```python
from build123d import *

# Parameters (mm, degrees)
SKETCH1_R           = 50
BOSS_EXTRUDE1_DEPTH = 10
SKETCH2_R           = 20
CUT_EXTRUDE1_DEPTH  = 74.484692283
CUT_EXTRUDE2_DEPTH  = 10
CUT_EXTRUDE3_DEPTH  = 10
CIRPATTERN1_COUNT   = 6
CIRPATTERN2_COUNT   = 6


with BuildPart() as part:
    # Sketch1 → Boss-Extrude1 (new, symmetric)
    with BuildSketch(Plane(origin=(0, 0, 0), x_dir=(1, 0, 0), z_dir=(0, 1, 0))):
        with Locations(Location((0, 0, 0), (0, 0, 270))):
            Circle(SKETCH1_R)
    extrude(amount=BOSS_EXTRUDE1_DEPTH, both=True)

    # Sketch2 → Cut-Extrude1 (cut, through all)
    with BuildSketch(Plane(origin=(0, 10, 0), x_dir=(1, 0, 0), z_dir=(0, 1, 0))):
        with Locations(Location((0, 0, 0), (0, 0, 270))):
            Circle(SKETCH2_R)
    extrude(amount=-CUT_EXTRUDE1_DEPTH, mode=Mode.SUBTRACT)

    # Sketch3 → Cut-Extrude2 (cut)
    with BuildSketch(Plane(origin=(0, 10, 0), x_dir=(1, 0, 0), z_dir=(0, 1, 0))):
        with BuildLine():
            Line((-7.5, 49.434299833), (-7.5, 18.540496218))
            ThreePointArc((-7.5, 18.540496218), (0, 20), (7.5, 18.540496218))
            Line((7.5, 18.540496218), (7.5, 49.434299833))
            ThreePointArc((7.5, 49.434299833), (0, 50), (-7.5, 49.434299833))
        make_face()
        with BuildLine():
            Line((39.061359474, 31.212340445), (12.306540723, 15.765438637))
            ThreePointArc((12.306540723, 15.765438637), (17.320508076, 10), (19.806540723, 2.77505758))
            Line((19.806540723, 2.77505758), (46.561359474, 18.221959388))
            ThreePointArc((46.561359474, 18.221959388), (43.301270189, 25), (39.061359474, 31.212340445))
        make_face()
        with BuildLine():
            Line((46.561359474, -18.221959388), (19.806540723, -2.77505758))
            ThreePointArc((19.806540723, -2.77505758), (17.320508076, -10), (12.306540723, -15.765438637))
            Line((12.306540723, -15.765438637), (39.061359474, -31.212340445))
            ThreePointArc((39.061359474, -31.212340445), (43.301270189, -25), (46.561359474, -18.221959388))
        make_face()
        with BuildLine():
            Line((7.5, -49.434299833), (7.5, -18.540496218))
            ThreePointArc((7.5, -18.540496218), (0, -20), (-7.5, -18.540496218))
            Line((-7.5, -18.540496218), (-7.5, -49.434299833))
            ThreePointArc((-7.5, -49.434299833), (0, -50), (7.5, -49.434299833))
        make_face()
        with BuildLine():
            Line((-39.061359474, -31.212340445), (-12.306540723, -15.765438637))
            ThreePointArc((-12.306540723, -15.765438637), (-17.320508076, -10), (-19.806540723, -2.77505758))
            Line((-19.806540723, -2.77505758), (-46.561359474, -18.221959388))
            ThreePointArc((-46.561359474, -18.221959388), (-43.301270189, -25), (-39.061359474, -31.212340445))
        make_face()
        with BuildLine():
            Line((-46.561359474, 18.221959388), (-19.806540723, 2.77505758))
            ThreePointArc((-19.806540723, 2.77505758), (-17.320508076, 10), (-12.306540723, 15.765438637))
            Line((-12.306540723, 15.765438637), (-39.061359474, 31.212340445))
            ThreePointArc((-39.061359474, 31.212340445), (-43.301270189, 25), (-46.561359474, 18.221959388))
        make_face()
    extrude(amount=-CUT_EXTRUDE2_DEPTH, mode=Mode.SUBTRACT)

    # Sketch4 → Cut-Extrude3 (cut)
    with BuildSketch(Plane(origin=(0, 10, 0), x_dir=(1, 0, 0), z_dir=(0, 1, 0))):
        with BuildLine():
            ThreePointArc((11, 48.774993593), (17.480362162, 30.322218565), (36.696416757, 33.961345633))
            ThreePointArc((36.696416757, 33.961345633), (24.971945946, 43.317455092), (11, 48.774993593))
        make_face()
    cut_extrude3 = extrude(amount=-CUT_EXTRUDE3_DEPTH, mode=Mode.SUBTRACT)

    # Sketch6 → Tap Drill for M10x1.0 Tap1 (revolve, cut)
    with BuildSketch(Plane(origin=(30, 10, 0), x_dir=(0, 0, 1), z_dir=(1, 0, 0))):
        Polygon((0, 0), (0, 72.703872786), (4.5, 70), (4.5, 0.025), (4.525, 0), align=None)
    tap_drill_for_m10x1_0_tap1 = revolve(axis=Axis((30, 16.35, 0), (0, -1, 0)), mode=Mode.SUBTRACT)

    # CirPattern1: Tap Drill for M10x1.0 Tap1 ×6 about axis
    cirpattern1_axis = Axis((0, 0, 0), (0, 1, 0))
    for i in range(1, CIRPATTERN1_COUNT):
        add(tap_drill_for_m10x1_0_tap1.rotate(cirpattern1_axis, i * 360 / CIRPATTERN1_COUNT), mode=Mode.SUBTRACT)

    # CirPattern2: Cut-Extrude3 ×6 about axis
    cirpattern2_axis = Axis((0, 0, 0), (0, 1, 0))
    for i in range(1, CIRPATTERN2_COUNT):
        add(cut_extrude3.rotate(cirpattern2_axis, i * 360 / CIRPATTERN2_COUNT), mode=Mode.SUBTRACT)


solid = part.part
```
Could you check a few things on this model? Use its own coordinates, in mm. A direction names the side the tool comes from. Coordinates: 2 decimals unless noted, no trailing zeros. Write each loop counter-clockwise with the first axis right and the second up, starting at its lowest first coordinate (ties: lowest second). Pieces come first, ordered by that corner, then holes. Notation, with made-up numbers: (50.25, 10) - (65.25, 10) arc R14 ccw to (65.25, 17) - close; hole circle Ø8 at (65.25, -2.5). An arc over 180 degrees is marked (long way). Use a Markdown table: item, result.
Q1. Thinking about a two-plate mould opening in X: for faces 4 (the cylindrical face through (-35, 5, 0)), 5 (the flat face through (23, 0, 37)), 6 (the cylindrical face through (17.779, 5.07, 30.153)), 7 (the flat face through (-20, 10, 29)), which applies, +X half, -X half, draft (parallel to the pull), parting line (faces both ways), or undercut?
Geometry check:
| item | result |
|---|---|
| face 4 | -X half |
| face 5 | undercut |
| face 6 | undercut |
| face 7 | draft |
Q2. Please list where these lines run through material, in increasing order: L1, parallel to X at y = -2.5, z = 0; L2, parallel to X at y = 8.25, z = -0.5; L3, parallel to Y at x = 2, z = 20.
Geometry check:
| item | result |
|---|---|
| L1 | x = -50 to -34.5, -25.5 to -20, 20 to 25.5, 34.5 to 50 |
| L2 | x = -35.01 to -34.47, -25.53 to -19.99, 19.99 to 25.53, 34.47 to 35.01 |
| L3 | y = -10 to 0 |
Q3. Imagine slicing it at B-B (z = -10). List the corners of the cut face in (x, y) for me, and give its area (3 significant figures).
Geometry check:
| item | result |
|---|---|
| outline | (-48.99, -10) - (-17.32, -10) - (-17.32, 0) - (-32.32, 0) - (-32.32, 10) - (-38.85, 10) - (-38.85, 0) - (-48.99, 0) - close; (17.32, -10) - (48.99, -10) - (48.99, 0) - (38.79, 0) - (38.79, 10) - (32.32, 10) - (32.32, 0) - (17.32, 0) - close |
| area | 763 mm2 |
Q4. Imagine slicing it at D-D (y = -3). List the corners of the cut face in (x, z) for me, and give its area (3 significant figures).
Geometry check:
| item | result |
|---|---|
| outline | circle Ø100 at (0, 0); hole circle Ø9 at (-30, 0); hole circle Ø40 at (0, 0); hole circle Ø9 at (-15, -25.98); hole circle Ø9 at (-15, 25.98); hole circle Ø9 at (15, -25.98); hole circle Ø9 at (15, 25.98); hole circle Ø9 at (30, 0) |
| area | 6,220 mm2 |
Q5. I'm going to push flat-ended pins straight in: pin 1 Ø2 at (x, z) = (-31.5, 4) entering from -Y; pin 2 Ø12 at (y, z) = (-3, -29) entering from -X; pin 3 Ø16.5 at (x, z) = (-18.5, 42) entering from +Y; pin 4 Ø5 at (y, z) = (3.5, -41) entering from -X. Where does each tip first touch, or does it pass through?
Geometry check:
| item | result |
|---|---|
| pin 1 | stops at y = -10 |
| pin 2 | stops at x = -44.4 |
| pin 3 | stops at y = 0 |
| pin 4 | stops at x = -10.81 |
Q6. Imagine slicing it at C-C (x = 15). Count the separate pieces of the cut face and the enclosed holes in it, and give its area (3 significant figures).
Geometry check:
| item | result |
|---|---|
| separate pieces | 4 |
| enclosed holes | 0 |
| area | 625 mm2 |
Q7. Imagine slicing it at A-A (x = 0). List the corners of the cut face in (y, z) for me, and give its area (3 significant figures).
Geometry check:
| item | result |
|---|---|
| outline | (-10, -50) - (0, -50) - (0, -20) - (-10, -20) - close; (-10, 20) - (0, 20) - (0, 50) - (-10, 50) - close |
| area | 600 mm2 |
Q8. Which directions (+Z, -Z, +X, -X, +Y, -Y) give clear straight access to the entire face, cutting with the end or side of a thin tool? Please do faces 1 (the cylindrical face through (35, 5, 0)), 2 (the flat face through (7.5, 5, -34)), 3 (the flat face through (29, 0, -17)).
Geometry check:
| item | result |
|---|---|
| face 1 | +X, +Y |
| face 2 | +Z, -Z, +Y |
| face 3 | +Y |
